Design review of the part built by this model. Coordinates are the model's own, in mm. A direction names the side the tool comes from. Give positions to 0.01 mm unless a question says otherwise; leave off trailing zeros. Write each loop counter-clockwise with the first axis right and the second up, starting at its lowest first coordinate (ties: lowest second). Pieces come first, ordered by that corner, then holes. Notation, with made-up numbers: M 7,0 L 63,0 A31 cw 63,32 Z; hole C 87,63.25 d2. An arc over 180 degrees is marked long. Answer in a Markdown table with one row per item.
```python
from build123d import *

# Parameters (mm, degrees)
BOSS_EXTRUDE1_DEPTH = 12.5


with BuildPart() as part:
    # Sketch4 → Boss-Extrude1 (new body)
    with BuildSketch(Plane.XY):
        Polygon((15, 32.102616066), (15, 29.909064249), (2, 29.909064249), (5.227521969, 38.776607979), (15.250051757, 50.72099386), (25.745438879, 63.228909169), (25.745438879, 44.908531455), align=None)
        Polygon((-2, 29.909064249), (-15, 29.909064249), (-15, 32.102616066), (-25.745438879, 44.908531455), (-25.745438879, 63.228909169), (-15.250051757, 50.72099386), (-5.227521969, 38.776607979), align=None)
        Polygon((-2, 29.909064249), (-2, 9.909064249), (2, 9.909064249), (2, 29.909064249), (15, 29.909064249), (15, 0), (-15, 0), (-15, 29.909064249), align=None)
    extrude(amount=BOSS_EXTRUDE1_DEPTH)


solid = part.part
```
1) Add section C-C (y = 59). Write out the cut boundary in (x, z).
Geometry says:
| item | result |
|---|---|
| outline | M -25.75,0 L -22.2,0 L -22.2,12.5 L -25.75,12.5 Z; M 22.2,0 L 25.75,0 L 25.75,12.5 L 22.2,12.5 Z |
2) The part is to be moulded in two halves that separate along X. For faces 1 (the face through (25.745, 54, 6)), 2 (the face through (-3.636, 34.405, 6.162)), 3 (the face through (-15, 16, 6)), 4 (the face through (6, 32, 0)), say which applies: released by +X, released by -X, zero draft, split by the parting line, or undercut.
Geometry says:
| item | result |
|---|---|
| face 1 | released by +X |
| face 2 | undercut |
| face 3 | released by -X |
| face 4 | zero draft |
3) Add section B-B (z = 5.75). Write out the cut boundary in (x, y).
Geometry says:
| item | result |
|---|---|
| outline | M -25.75,44.91 L -15,32.1 L -15,0 L 15,0 L 15,32.1 L 25.75,44.91 L 25.75,63.23 L 5.23,38.78 L 2,29.91 L 2,9.91 L -2,9.91 L -2,29.91 L -5.23,38.78 L -25.75,63.23 Z |
4) Add section D-D (x = 4). Write out the cut boundary in (y, z).
Geometry says:
| item | result |
|---|---|
| outline | M 0,0 L 35.4,0 L 35.4,12.5 L 0,12.5 Z |
5) For faces 5 (the face through (0, 0, 6)), 6 (the face through (0, 9.909, 6)), 7 (the face through (15, 16, 6)), list the 3-axis set-ups (+Z, -Z, +X, -X, +Y, -Y) from which the entire face can be reached by the end or side of a thin tool; tool diameter is ignored.
Geometry says:
| item | result |
|---|---|
| face 5 | +Z, -Z, +X, -X, -Y |
| face 6 | +Z, -Z, +Y |
| face 7 | +Z, -Z, +X, -Y |
6) Insertion check: P1, Ø1, axis at x = 1.5, z = 8.5, coming from the -Y side; P2, Ø2, axis at x = 0, z = 3.5, coming from the +Y side; P3, Ø4, axis at y = 35.5, z = 3, coming from the +X side; P4, Ø1.5, axis at x = 8, z = 5.5, coming from the +Y side. Each pin has a flat end and moves straight along its axis. Give the tip position at first contact, or say it passes through.
Geometry says:
| item | result |
|---|---|
| P1 | y = 0 |
| P2 | y = 9.91 |
| P3 | x = 19.53 |
| P4 | y = 42.97 |
7) To check wall thickness, follow probe 1 along X at (y, z) = (18.5, 3); probe 2 along Y at (x, z) = (-0.5, 7.75); probe 3 along X at (y, z) = (8, 9). State the ranges of each line that lie inside material, in increasing order. Write a range as [from, to].
Geometry says:
| item | result |
|---|---|
| probe 1 | [-15, -2], [2, 15] |
| probe 2 | [0, 9.91] |
| probe 3 | [-15, 15] |
8) Add section A-A (y = 21.5). Write out the cut boundary in (x, z), and give its area (3 significant figures).
Geometry says:
| item | result |
|---|---|
| outline | M -15,0 L -2,0 L -2,12.5 L -15,12.5 Z; M 2,0 L 15,0 L 15,12.5 L 2,12.5 Z |
| area | 325 mm^2 |
